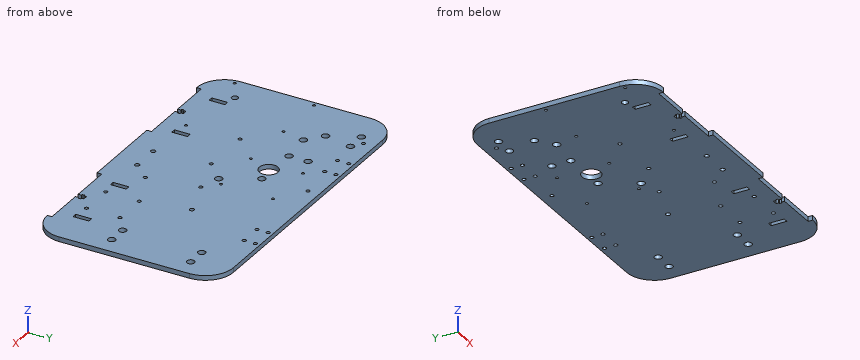
```python
from build123d import *

# Parameters (mm, degrees)
SALIENTE_EXTRUIR1_DEPTH = 5
CROQUIS2_R              = 4
CORTAR_EXTRUIR4_DEPTH   = 10
CROQUIS3_R              = 2
CROQUIS3_R_2            = 10
CROQUIS3_R_3            = 4.05
CORTAR_EXTRUIR5_DEPTH   = 10
CROQUIS5_R              = 1.5
CORTAR_EXTRUIR6_DEPTH   = 10
CROQUIS6_R              = 2
CORTAR_EXTRUIR7_DEPTH   = 10
CROQUIS8_R              = 2
CORTAR_EXTRUIR8_DEPTH   = 10
CROQUIS9_R              = 3.5
CROQUIS9_R_2            = 1.5
CROQUIS9_R_3            = 2.5
CROQUIS9_R_4            = 2
CORTAR_EXTRUIR9_DEPTH   = 10
CROQUIS10_W             = 93.333333333
CROQUIS10_H             = 5
CORTAR_EXTRUIR10_DEPTH  = 10
CORTAR_EXTRUIR14_DEPTH  = 5
CROQUIS13_W             = 5
CROQUIS13_H             = 17
CORTAR_EXTRUIR15_DEPTH  = 5
CROQUIS14_R             = 2.5
CORTAR_EXTRUIR16_DEPTH  = 10


with BuildPart() as part:
    # Croquis1 → Saliente-Extruir1 (new body)
    with BuildSketch(Plane.XY):
        with BuildLine():
            Line((30, 0), (310, 0))
            ThreePointArc((310, 0), (331.213203436, 8.786796564), (340, 30))
            Line((340, 30), (340, 170))
            ThreePointArc((340, 170), (331.213203436, 191.213203436), (310, 200))
            Line((310, 200), (30, 200))
            ThreePointArc((30, 200), (8.786796564, 191.213203436), (0, 170))
            Line((0, 170), (0, 30))
            ThreePointArc((0, 30), (8.786796564, 8.786796564), (30, 0))
        make_face()
    extrude(amount=SALIENTE_EXTRUIR1_DEPTH)

    # Croquis2 → Cortar-Extruir4 (cut)
    with BuildSketch(Plane(origin=(0, 0, 5), x_dir=(-1, 0, 0), z_dir=(0, 0, -1))):
        with Locations((-55.5, 180)):
            Circle(CROQUIS2_R)
        with Locations((-35, 180)):
            Circle(CROQUIS2_R)
        with Locations((-100, 160)):
            Circle(CROQUIS2_R)
        with Locations((-100, 139.5)):
            Circle(CROQUIS2_R)
        with Locations((-299.5, 160)):
            Circle(CROQUIS2_R)
        with Locations((-320, 160)):
            Circle(CROQUIS2_R)
        with Locations((-320, 75)):
            Circle(CROQUIS2_R)
        with Locations((-299.5, 75)):
            Circle(CROQUIS2_R)
        with Locations((-150, 139)):
            Circle(CROQUIS2_R)
        with Locations((-170, 104)):
            Circle(CROQUIS2_R)
        with Locations((-50, 150)):
            Circle(CROQUIS2_R)
    extrude(amount=CORTAR_EXTRUIR4_DEPTH, mode=Mode.SUBTRACT)

    # Croquis3 → Cortar-Extruir5 (cut)
    with BuildSketch(Plane(origin=(0, 0, 0), x_dir=(-1, 0, 0), z_dir=(0, 0, -1))):
        with Locations((-148.85, 83.84)):
            Circle(CROQUIS3_R)
        with Locations((-94.85, 83.84)):
            Circle(CROQUIS3_R)
        with Locations((-44.85, 187.84)):
            Circle(CROQUIS3_R)
        with Locations((-148.85, 187.84)):
            Circle(CROQUIS3_R)
        with Locations((-131.95, 135.84)):
            Circle(CROQUIS3_R_2)
        with Locations((-66.85, 135.84)):
            Circle(CROQUIS3_R_3)
    extrude(amount=-CORTAR_EXTRUIR5_DEPTH, mode=Mode.SUBTRACT)

    # Croquis5 → Cortar-Extruir6 (cut)
    with BuildSketch(Plane(origin=(0, 0, 0), x_dir=(-1, 0, 0), z_dir=(0, 0, -1))):
        with Locations((-178, 167)):
            Circle(CROQUIS5_R)
        with Locations((-122, 111)):
            Circle(CROQUIS5_R)
        with Locations((-122, 167)):
            Circle(CROQUIS5_R)
        with Locations((-178, 111)):
            Circle(CROQUIS5_R)
    extrude(amount=-CORTAR_EXTRUIR6_DEPTH, mode=Mode.SUBTRACT)

    # Croquis6 → Cortar-Extruir7 (cut)
    with BuildSketch(Plane.XY.offset(5)):
        with Locations((244, 61)):
            Circle(CROQUIS6_R)
        with Locations((280, 61)):
            Circle(CROQUIS6_R)
        with Locations((244, 25)):
            Circle(CROQUIS6_R)
        with Locations((280, 25)):
            Circle(CROQUIS6_R)
    extrude(amount=-CORTAR_EXTRUIR7_DEPTH, mode=Mode.SUBTRACT)

    # Croquis8 → Cortar-Extruir8 (cut)
    with BuildSketch(Plane.XY.offset(5)):
        with Locations((236, 195)):
            Circle(CROQUIS8_R)
        with Locations((236, 183)):
            Circle(CROQUIS8_R)
        with Locations((260, 183)):
            Circle(CROQUIS8_R)
        with Locations((260, 195)):
            Circle(CROQUIS8_R)
        with Locations((85, 195)):
            Circle(CROQUIS8_R)
        with Locations((85, 183)):
            Circle(CROQUIS8_R)
        with Locations((109, 183)):
            Circle(CROQUIS8_R)
        with Locations((109, 195)):
            Circle(CROQUIS8_R)
    extrude(amount=-CORTAR_EXTRUIR8_DEPTH, mode=Mode.SUBTRACT)

    # Croquis9 → Cortar-Extruir9 (cut)
    with BuildSketch(Plane(origin=(0, 0, 0), x_dir=(-1, 0, 0), z_dir=(0, 0, -1))):
        with Locations((-29.01, 40.656502357)):
            Circle(CROQUIS9_R)
        with Locations((-62.080404779, 111.910005093)):
            Circle(CROQUIS9_R_2)
        with Locations((-4.98, 111.910005093)):
            Circle(CROQUIS9_R_2)
        with Locations((-97.280894834, 27.160005093)):
            Circle(CROQUIS9_R_2)
        with Locations((-4.98, 26.56)):
            Circle(CROQUIS9_R_2)
        with Locations((-233.296749654, 111.494889841)):
            Circle(CROQUIS9_R_3)
        with Locations((-201.8, 43.4)):
            Circle(CROQUIS9_R_4)
        with Locations((-192.05, 97.413240345)):
            Circle(CROQUIS9_R_4)
    extrude(amount=-CORTAR_EXTRUIR9_DEPTH, mode=Mode.SUBTRACT)

    # Croquis10 → Cortar-Extruir10 (cut)
    with BuildSketch(Plane.XY.offset(5)):
        with Locations((76.666666667, 2.5)):
            Rectangle(CROQUIS10_W, CROQUIS10_H)
        with Locations((263.333333334, 2.5)):
            Rectangle(CROQUIS10_W, CROQUIS10_H)
    extrude(amount=-CORTAR_EXTRUIR10_DEPTH, mode=Mode.SUBTRACT)

    # Croquis12 → Cortar-Extruir14 (cut)
    with BuildSketch(Plane.XY.offset(5)):
        Polygon((74.166666667, 5), (74.166666667, 8.5), (72.666666667, 8.5), (72.666666667, 11.3), (74.166666667, 11.3), (74.166666667, 14), (79.166666667, 14), (79.166666667, 11.3), (80.666666667, 11.3), (80.666666667, 8.5), (79.166666667, 8.5), (79.166666667, 5), align=None)
        Polygon((260.833333333, 11.3), (260.833333333, 14), (265.833333333, 14), (265.833333333, 11.3), (267.333333333, 11.3), (267.333333333, 8.5), (265.833333333, 8.5), (265.833333333, 5), (260.833333333, 5), (260.833333333, 8.5), (259.333333333, 8.5), (259.333333333, 11.3), align=None)
    extrude(amount=-CORTAR_EXTRUIR14_DEPTH, mode=Mode.SUBTRACT)

    # Croquis13 → Cortar-Extruir15 (cut)
    with BuildSketch(Plane.XY.offset(5)):
        with Locations((42.5, 30.5)):
            Rectangle(CROQUIS13_W, CROQUIS13_H)
        with Locations((112.5, 30.5)):
            Rectangle(CROQUIS13_W, CROQUIS13_H)
        with Locations((227.5, 30.5)):
            Rectangle(CROQUIS13_W, CROQUIS13_H)
        with Locations((297.5, 30.5)):
            Rectangle(CROQUIS13_W, CROQUIS13_H)
    extrude(amount=-CORTAR_EXTRUIR15_DEPTH, mode=Mode.SUBTRACT)

    # Croquis14 → Cortar-Extruir16 (cut)
    with BuildSketch(Plane.XY.offset(5)):
        with Locations((155, 25)):
            Circle(CROQUIS14_R)
        with Locations((185, 25)):
            Circle(CROQUIS14_R)
    extrude(amount=-CORTAR_EXTRUIR16_DEPTH, mode=Mode.SUBTRACT)


solid = part.part
```
Source: CAD feature listing. Evaluate the final solid. Frame: model axes, mm. Coordinates: 2 decimals unless noted, no trailing zeros. Order: outer loops, then holes, each group sorted by start corner. A loop starts at its lowest first (then second) coordinate and runs counter-clockwise, first axis right, second up. Notation, with made-up numbers: (-28.75, 6.5) - (-21.75, 6.5) arc R16 ccw to (-21.75, 19.5) - close; hole circle Ø3 at (51, 48.25). An arc over 180 degrees is marked (long way). One line per item, written item: value.
1) Ray query, line 1 (X direction, y = 167, z = 1.1); line 2 (Y direction, x = 280, z = 4.15); line 3 (Y direction, x = 260, z = 1.6). Return the intervals inside material, ascending. Write a range as [from, to].
Computed values:
line 1: x = [0, 120.5], [123.5, 176.5], [179.5, 340]
line 2: y = [5, 23], [27, 59], [63, 200]
line 3: y = [5, 8.5], [11.3, 181], [185, 193], [197, 200]
2) Cut plane C-C on z = 4. State how many separate pieces and enclosed holes the cut face has, plus the area to 3 significant figures.
Computed values:
separate pieces: 1
enclosed holes: 47
area: 64,500 mm^2
3) Cut plane B-B on x = 131.95. Output: boundary loops of the cut face in (y, z).
Computed values:
outline: (0, 0) - (125.84, 0) - (125.84, 5) - (0, 5) - close; (145.84, 0) - (200, 0) - (200, 5) - (145.84, 5) - close
4) Contact query for flat-ended pins moving along their axis: pin 1 (1 mm diameter, centred on x = 94, y = 157, fed in from -Z); pin 2 (3.5 mm diameter, centred on x = 244, y = 25, fed in from +Z); pin 3 (2.5 mm diameter, centred on y = 3, z = 1.5, fed in from +X); pin 4 (1.5 mm diameter, centred on x = 297.5, z = 3, fed in from -Y). Output: stop coordinate, or through.
Computed values:
pin 1: stops at z = 0
pin 2: passes through
pin 3: stops at x = 325.39
pin 4: stops at y = 5
5) Cut plane A-A on y = 160. Output: boundary loops of the cut face in (x, z), plus the area to 3 significant figures.
Computed values:
outline: (0, 0) - (96, 0) - (96, 5) - (0, 5) - close; (104, 0) - (295.5, 0) - (295.5, 5) - (104, 5) - close; (303.5, 0) - (316, 0) - (316, 5) - (303.5, 5) - close; (324, 0) - (340, 0) - (340, 5) - (324, 5) - close
area: 1,580 mm^2
6) Cut plane D-D on x = 170.5. Output: boundary loops of the cut face in (y, z), plus the area to 3 significant figures.
Computed values:
outline: (0, 0) - (100.03, 0) - (100.03, 5) - (0, 5) - close; (107.97, 0) - (200, 0) - (200, 5) - (107.97, 5) - close
area: 960 mm^2
